Geometry check sheet. Reference: the model listing, model coordinates, mm. A direction names the side the tool comes from. Round coordinates to 2 decimals unless told otherwise and drop trailing zeros. Write each loop counter-clockwise with the first axis right and the second up, starting at its lowest first coordinate (ties: lowest second). Pieces come first, ordered by that corner, then holes. Notation, with made-up numbers: (21, 28.25) - (26, 28.25) arc R15 cw to (26, 40.25) - close; hole circle Ø11 at (70, -3). An arc over 180 degrees is marked (long way). Return JSON: item names as keys, results as strings.
Autodesk Fusion 360 part; units mm, degrees
sketch "Sketch1" plane through (0, 0, 0) normal (0, 0, 1) x (1, 0, 0)
  line L0 (0, 0) -> (20, 0)
  line L1 (20, 0) -> (20, 15)
  line L2 (20, 15) -> (0, 15)
  line L3 (0, 15) -> (0, 0)
  dimension "d1" = 20
  dimension "d2" = 15
extrude "Extrude1" add sketch "Sketch1" along normal blind 4
sketch "Sketch2" plane through (0, 0, 4) normal (0, 0, 1) x (-1, 0, 0)
  line L0 (0, -15) -> (0, 0)
  line L1 (0, 0) -> (-20, 0)
  line L2 (-20, 0) -> (-20, -15)
  line L3 (-20, -15) -> (0, -15)
  point P0 (-5, -11)
  point P1 (-15, -11)
  point P2 (-15, -3.5)
  point P3 (-5, -3.5)
  dimension "d5" = 10
  dimension "d6" = 10
  dimension "d7" = 5
  dimension "d8" = 5
  dimension "d9" = 4
  dimension "d10" = 7.5
hole "Hole1" at (5, 11, 4) at (15, 11, 4) at (15, 3.5, 4) at (5, 3.5, 4) direction (0, 0, -1) diameter 3.3 depth 11 tip angle 118
extrude "Extrude2" cut 1 faces at (13.3333, 15, 1.3333) along direction (0, -1, 0) blind 0.3
extrude "Extrude3" add 1 faces at (6.6667, 0, 1.3333) along direction (0, -1, 0) blind 0.3
extrude "Extrude4" add 1 faces at (6.6667, -0.3, 1.3333) along direction (0, -1, 0) blind 5
sketch "Sketch3" plane through (0, 0, 4) normal (0, 0, 1) x (-1, 0, 0)
  line L0 (-20, -14.7) -> (0, -14.7)
  line L1 (0, -14.7) -> (0, 5.3)
  line L2 (0, 5.3) -> (-20, 5.3)
  line L3 (-20, 5.3) -> (-20, -14.7)
  circle A0 centre (-5, -3.5) radius 1.65
  circle A1 centre (-15, -11) radius 1.65
  circle A2 centre (-5, -11) radius 1.65
  circle A3 centre (-15, -3.5) radius 1.65
  line L4 (0, 5.3) -> (-20, 5.3)
  line L5 (-20, 5.3) -> (-20, 0.3)
  line L6 (-20, 0.3) -> (0, 0.3)
  line L7 (0, 0.3) -> (0, 5.3)
  dimension "d20" = 5
extrude "Extrude5" add sketch "Sketch3" along normal blind 20 contours L1 L2 L3 L4 L5 L6 L7
sketch "Sketch4" plane through (0, -0.3, 0) normal (0, 1, 0) x (-1, 0, 0)
  line L0 (-20, 4) -> (0, 4)
  line L1 (0, 4) -> (0, 24)
  line L2 (0, 24) -> (-20, 24)
  line L3 (-20, 24) -> (-20, 4)
  line L4 (0, 0) -> (-20, 0)
  point P0 (-10, 15.125)
  dimension "d23" = 15.125
  dimension "d24" = 10
hole "Hole2" at (10, -0.3, 15.125) direction (0, -1, 0) diameter 6.5 depth 11 tip angle 118
sketch "Sketch5" plane through (0, -0.3, 0) normal (0, 1, 0) x (-1, 0, 0)
  circle A0 centre (-10, 15.125) radius 3.25
  line L0 (-20, 4) -> (0, 4)
  line L1 (0, 4) -> (0, 24)
  line L2 (0, 24) -> (-20, 24)
  line L3 (-20, 24) -> (-20, 4)
  circle A1 centre (-10, 15.125) radius 3.75
  dimension "d28" = 7.5
extrude "Extrude6" cut sketch "Sketch5" against normal blind 12.823 contours A1
sketch "Sketch6" plane through (0, -5.3, 0) normal (0, -1, 0) x (1, 0, 0)
  circle A0 centre (10, 15.125) radius 3.75
  line L0 (0, 0) -> (20, 0)
  line L1 (20, 0) -> (20, 24)
  line L2 (20, 24) -> (0, 24)
  line L3 (0, 24) -> (0, 0)
  circle A1 centre (10, 15.125) radius 6.5
  dimension "d31" = 13
extrude "Extrude7" cut sketch "Sketch6" against normal blind 68.492 contours A1
extrude "Extrude8" add 1 faces at (9.8381, -5.3, 2.8811) along direction (0, -1, 0) blind 2
equation "d9 = 2.3 mm + 1.7 mm"
equation "d23 = 18.3 mm - ( 6.35 / 2 ) * 1 mm"
(1) Gauge pin test, flat ends, axial feed: pin 1 (3 mm diameter, centred on x = 7, z = 19.5, fed in from +Y); pin 2 (6 mm diameter, centred on x = 13, y = 5, fed in from +Z). Record the tip position at first contact, or that the pin passes through.
Response values:
{"pin 1": "stops at y = -0.3", "pin 2": "stops at z = 4"}
(2) Material ranges on line 1 along X through (y, z) = (11, 2.85); line 2 along Y through (x, z) = (5, 1.85); line 3 along Z through (x, y) = (10, -5) (3 decimals), recorded low to high. Write a range as [from, to].
Response values:
{"line 1": "x = [0, 3.35], [6.65, 13.35], [16.65, 20]", "line 2": "y = [-7.3, 1.85], [5.15, 9.35], [12.65, 14.7]", "line 3": "z = [0, 8.625], [21.625, 24]"}
(3) Access from +Z, -Z, +X, -X, +Y, -Y to the whole of each face (thin tool, end or side, straight path). Record for faces 1 (the face through (10, 7, 4)), 2 (the face through (13.885, 4.716, 1.972)).
Response values:
{"face 1": "+Z, +X, -X, +Y", "face 2": "+Z, -Z"}
(4) Section check C-C, the plane z = 15.75. Enter the section's corners in (x, y), plus the area to 3 significant figures.
Response values:
{"outline": "(0, -7.3) - (3.53, -7.3) - (3.53, -0.3) - (0, -0.3) - close; (16.47, -7.3) - (20, -7.3) - (20, -0.3) - (16.47, -0.3) - close", "area": "49.4 mm^2"}
(5) Section check D-D, the plane x = 5. Enter the section's corners in (y, z).
Response values:
{"outline": "(-7.3, 0) - (1.85, 0) - (1.85, 4) - (-0.3, 4) - (-0.3, 10.97) - (-7.3, 10.97) - close; (-7.3, 19.28) - (-0.3, 19.28) - (-0.3, 24) - (-7.3, 24) - close; (5.15, 0) - (9.35, 0) - (9.35, 4) - (5.15, 4) - close; (12.65, 0) - (14.7, 0) - (14.7, 4) - (12.65, 4) - close"}
(6) Release check for a two-part mould opening along Y. For faces 3 (the face through (5.632, 9.476, 1.972)), 4 (the face through (13.61, 10.11, 1.97)), 5 (the face through (10, -7.3, 6)), 6 (the face through (0, -1, 10)) record: pulls with the +Y half, pulls with the -Y half, needs draft (parallel to the pull), parting line crosses it, or undercut.
Response values:
{"face 3": "undercut", "face 4": "undercut", "face 5": "pulls with the -Y half", "face 6": "needs draft"}
(7) Section check B-B, the plane y = 3.5. Enter the section's corners in (x, z), plus the area to 3 significant figures.
Response values:
{"outline": "(0, 0) - (3.35, 0) - (3.35, 4) - (0, 4) - close; (6.65, 0) - (13.35, 0) - (13.35, 4) - (6.65, 4) - close; (16.65, 0) - (20, 0) - (20, 4) - (16.65, 4) - close", "area": "53.6 mm^2"}
(8) Section check A-A, the plane x = 10. Enter the section's corners in (y, z) (3 decimals), plus the area to 3 significant figures.
Response values:
{"outline": "(-7.3, 0) - (14.7, 0) - (14.7, 4) - (-0.3, 4) - (-0.3, 8.625) - (-7.3, 8.625) - close; (-7.3, 21.625) - (-0.3, 21.625) - (-0.3, 24) - (-7.3, 24) - close", "area": "137 mm^2"}
